Build history of the part. All positions in model axes, mm. Give positions to 0.01 mm unless a question says otherwise; leave off trailing zeros. Order: outer loops, then holes, each group sorted by start corner. A loop starts at its lowest first (then second) coordinate and runs counter-clockwise, first axis right, second up. Notation, with made-up numbers: (19, -35.5) - (37, -35.5) arc R29 ccw to (37, 3.5) - close; hole circle Ø10 at (18, -9). An arc over 180 degrees is marked (long way). Use a Markdown table: item, result.
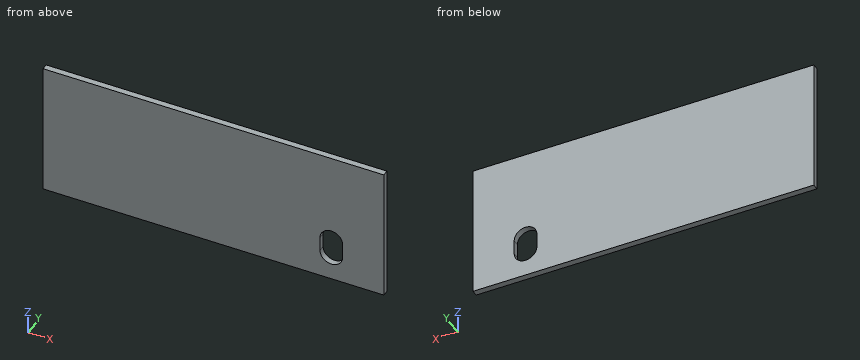
Autodesk Inventor part; units mm, degrees
ref_plane "YZ Plane" through (0, 0, 0) normal (1, 0, 0) x (0, 1, 0)
ref_plane "XZ Plane" through (0, 0, 0) normal (0, 1, 0) x (-1, 0, 0)
ref_plane "XY Plane" through (0, 0, 0) normal (0, 0, 1) x (1, 0, 0)
sketch "Skizze1" plane through (0, 0, 0) normal (0, 1, 0) x (-1, 0, 0)
  line L0 (0, 0) -> (-165.5, 0)
  line L1 (-165.5, 0) -> (-165.5, -65.5)
  line L2 (-165.5, -65.5) -> (0, -65.5)
  line L3 (0, -65.5) -> (0, 0)
  line L4 (-134.5, -45) -> (-134.5, -52)
  line L5 (-145.5, -52) -> (-145.5, -45)
  arc A0 (-145.5, -52) -> (-134.5, -52) centre (-140, -52) ccw
  arc A1 (-134.5, -45) -> (-145.5, -45) centre (-140, -45) ccw
  dimension "d0" = 165.5
  dimension "d1" = 65.5
  dimension "d8" = 11
  dimension "d9" = 7
  dimension "d10" = 13.5
  dimension "d11" = 20
extrude "Extrusion1" add sketch "Skizze1" along normal blind 3
properties part number "wood_front"
1) Slice it at B-B (z = -49). Write the cut outline in (x, y).
Computed:
| item | result |
|---|---|
| outline | (0, 0) - (134.5, 0) - (134.5, 3) - (0, 3) - close; (145.5, 0) - (165.5, 0) - (165.5, 3) - (145.5, 3) - close |
2) Pin check, flat tip, straight feed: P1, Ø1, axis at x = 121, y = 1.5, coming from the +Z side. Stop position of the tip, or through.
Computed:
| item | result |
|---|---|
| P1 | stops at z = 0 |
3) Slice it at C-C (y = 2.4). Write the cut outline in (x, z).
Computed:
| item | result |
|---|---|
| outline | (0, -65.5) - (165.5, -65.5) - (165.5, 0) - (0, 0) - close; hole (134.5, -52) arc R5.5 ccw to (145.5, -52) - (145.5, -45) arc R5.5 ccw to (134.5, -45) - close |
4) Slice it at A-A (x = 140). Write the cut outline in (y, z).
Computed:
| item | result |
|---|---|
| outline | (0, -65.5) - (3, -65.5) - (3, -57.5) - (0, -57.5) - close; (0, -39.5) - (3, -39.5) - (3, 0) - (0, 0) - close |
5) Wall check: line 1 (Z direction, x = 145, y = 0.35); line 2 (Z direction, x = 142.5, y = 2.4); line 3 (X direction, y = 1.95, z = -54). Give the ranges that are in metal, low to high. Write a range as from..to.
Computed:
| item | result |
|---|---|
| line 1 | z = -65.5..-54.29, -42.71..0 |
| line 2 | z = -65.5..-56.9, -40.1..0 |
| line 3 | x = 0..134.88, 145.12..165.5 |
